from build123d import *

# Parameters (mm, degrees)
SKETCH1_R           = 3.25
BOSS_EXTRUDE1_DEPTH = 5
SKETCH2_R           = 2.075
BOSS_EXTRUDE2_DEPTH = 5
FILLET1_R           = 3


with BuildPart() as part:
    # Sketch1 → Boss-Extrude1 (new body)
    with BuildSketch(Plane(origin=(0, 0, 0), x_dir=(1, 0, 0), z_dir=(0, 1, 0))):
        Polygon((-59.15, -15), (-82.443714059, -101.933324366), (-63.125197533, -107.109705268), (-39.831483474, -20.176380902), (-39.15, -17.633049952), (-39.15, -15), (-39.15, 15), (-59.15, 15), align=None)
        with Locations((-49.15, 0)):
            Circle(SKETCH1_R, mode=Mode.SUBTRACT)
    extrude(amount=BOSS_EXTRUDE1_DEPTH)

    # Sketch2 → Boss-Extrude2 (add)
    with BuildSketch(Plane.XZ):
        Polygon((-14.15, -7.5), (-14.15, 7.5), (-27.15, 7.5), (-33.15, 7.5), (-39.15, 7.5), (-39.15, -7.5), align=None)
        with Locations((-33.15, 0)):
            Circle(SKETCH2_R, mode=Mode.SUBTRACT)
        with Locations((-27.15, 0)):
            Circle(SKETCH2_R, mode=Mode.SUBTRACT)
        with Locations((-21.15, 0)):
            Circle(SKETCH2_R, mode=Mode.SUBTRACT)
    extrude(amount=-BOSS_EXTRUDE2_DEPTH)

    # Fillet1
    fillet1_edges = [part.edges().sort_by_distance(p)[0] for p in [
        (-39.15, 2.5, 17.633049952),
        (-63.125197533, 2.5, 107.109705268),
        (-82.443714059, 2.5, 101.933324366),
        (-59.15, 2.5, 15),
        (-59.15, 2.5, -15),
        (-39.15, 2.5, -15),
        (-14.15, 2.5, -7.5),
        (-39.15, 2.5, -7.5),
        (-39.15, 2.5, 7.5),
        (-14.15, 2.5, 7.5),
    ]]
    fillet(fillet1_edges, radius=FILLET1_R)


solid = part.part
Source: CAD feature listing. Evaluate the final solid. Frame: model axes, mm. A direction names the side the tool comes from. Give positions to 0.01 mm unless a question says otherwise; leave off trailing zeros. Write each loop counter-clockwise with the first axis right and the second up, starting at its lowest first coordinate (ties: lowest second). Pieces come first, ordered by that corner, then holes. Notation, with made-up numbers: M 72.5,-36 L 96.5,-36 A18 cw 96.5,-5 Z; hole C 23.25,4 d2. An arc over 180 degrees is marked long. Return JSON: item names as keys, results as strings. Group by question number.
1) Cut plane B-B, the plane z = 0. Output: boundary loops of the cut face in (x, y) (3 decimals).
2) Draft query along Z for faces 5 (the face through (-72.879, 2.465, 104.496)), 6 (the face through (-35.223, 2.465, 0.091)), 7 (the face through (-38.29, 2.54, -8.4)). Return one class per face: released by +Z, released by -Z, zero draft, split by the parting line, or undercut.
3) Set-up query: faces 1 (the face through (-14.15, 2, 0)), 2 (the face through (-39.15, 2, 14)), 3 (the face through (-59.15, 2, 1)), 4 (the face through (-27, 2, -7.5)). Return all of +Z, -Z, +X, -X, +Y, -Y with unobstructed straight access to the full face (end or side cutting, diameter ignored); none if empty.
4) Ray query, L1, parallel to Z at x = -21.15, y = 2.1 (3 decimals); L2, parallel to X at y = 4.45, z = 1.5; L3, parallel to Z at x = -29.5, y = 1.6. Return the intervals inside material, ascending.
5) Cut plane C-C, the plane y = 3.3. Give the number of separate pieces and of enclosed holes in the cut face, then the cut area to 3 significant figures.
6) Cut plane A-A, the plane x = -27.15. Output: boundary loops of the cut face in (y, z) (3 decimals), then the cut area to 4 significant figures.
7) First-contact query: pin 1 Ø2.5 at (x, y) = (-25, 3) entering from -Z; pin 2 Ø5 at (x, z) = (-27.15, 0) entering from -Y; pin 3 Ø1.6 at (y, z) = (3.5, -11.5) entering from +X. Flat tips, straight axial feed; report the tip coordinate or a pass-through.
8) Cut plane D-D, the plane x = -48.5. Output: boundary loops of the cut face in (y, z), then the cut area to 3 significant figures.
Data:
{
 "1": {"outline": "M -59.15,0 L -52.4,0 L -52.4,5 L -59.15,5 Z; M -45.9,0 L -35.225,0 L -35.225,5 L -45.9,5 Z; M -31.075,0 L -29.225,0 L -29.225,5 L -31.075,5 Z; M -25.075,0 L -23.225,0 L -23.225,5 L -25.075,5 Z; M -19.075,0 L -14.15,0 L -14.15,5 L -19.075,5 Z"},
 "2": {"face 5": "released by +Z", "face 6": "undercut", "face 7": "released by -Z"},
 "3": {"face 1": "+Z, -Z, +X, +Y, -Y", "face 2": "+Z, +X, +Y, -Y", "face 3": "-Z, -X, +Y, -Y", "face 4": "-Z, +X, +Y, -Y"},
 "4": {"L1": "z = -7.5 to -2.075, 2.075 to 7.5", "L2": "x = -59.15 to -52.03, -46.27 to -34.58, -31.72 to -28.58, -25.72 to -22.58, -19.72 to -14.15", "L3": "z = -7.5 to 7.5"},
 "5": {"separate pieces": "1", "enclosed holes": "4", "area": "2,750 mm²"},
 "6": {"outline": "M 0,-7.5 L 5,-7.5 L 5,-2.075 L 0,-2.075 Z; M 0,2.075 L 5,2.075 L 5,7.5 L 0,7.5 Z", "area": "54.25 mm²"},
 "7": {"pin 1": "stops at z = -7.5", "pin 2": "stops at y = 0", "pin 3": "stops at x = -39.15"},
 "8": {"outline": "M 0,-15 L 5,-15 L 5,-3.18 L 0,-3.18 Z; M 0,3.18 L 5,3.18 L 5,52.53 L 0,52.53 Z", "area": "306 mm²"}
}
